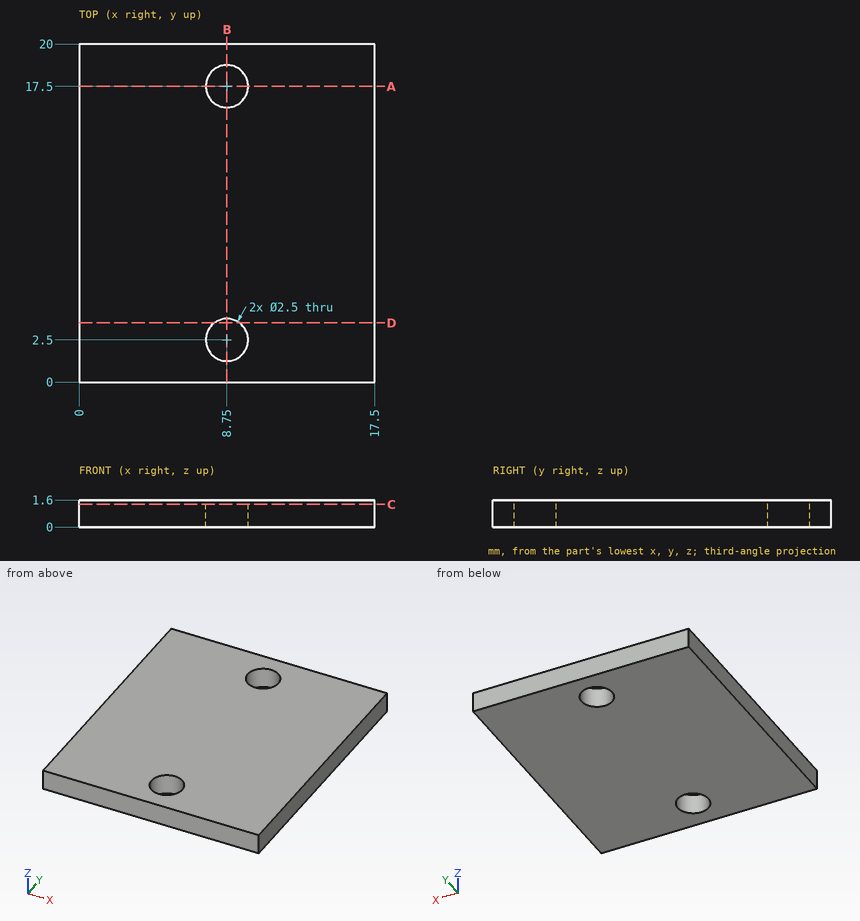
The drawing under review shows one solid part. Ordinate dimensions are in mm from its lowest x, y, z. Give positions to 0.01 mm unless a question says otherwise; leave off trailing zeros. Write each loop counter-clockwise with the first axis right and the second up, starting at its lowest first coordinate (ties: lowest second). Pieces come first, ordered by that corner, then holes.
1. Add section B-B, the plane x = 8.75. Write out the cut boundary in (y, z), plus the area to 3 significant figures.
2. Add section D-D, the plane y = 3.5. Write out the cut boundary in (x, z).
3. Wall thickness on L1, parallel to Y at x = 8.75, z = 0.75; L2, parallel to X at y = 17.5, z = 0.55; L3, parallel to Y at x = 8.25, z = 0.95: over which ranges is each line inside the solid? List them lowest first.
4. Add section C-C, the plane z = 1.35. Write out the cut boundary in (x, y).
5. Add section A-A, the plane y = 17.5. Write out the cut boundary in (x, z), plus the area to 3 significant figures.
Worked answers:
1. outline: (0, 0) - (1.25, 0) - (1.25, 1.6) - (0, 1.6) - close; (3.75, 0) - (16.25, 0) - (16.25, 1.6) - (3.75, 1.6) - close; (18.75, 0) - (20, 0) - (20, 1.6) - (18.75, 1.6) - close
1. area: 24.0 mm2
2. outline: (0, 0) - (8, 0) - (8, 1.6) - (0, 1.6) - close; (9.5, 0) - (17.5, 0) - (17.5, 1.6) - (9.5, 1.6) - close
3. L1: y = 0 to 1.25, 3.75 to 16.25, 18.75 to 20
3. L2: x = 0 to 7.5, 10 to 17.5
3. L3: y = 0 to 1.35, 3.65 to 16.35, 18.65 to 20
4. outline: (0, 0) - (17.5, 0) - (17.5, 20) - (0, 20) - close; hole circle Ø2.5 at (8.75, 2.5); hole circle Ø2.5 at (8.75, 17.5)
5. outline: (0, 0) - (7.5, 0) - (7.5, 1.6) - (0, 1.6) - close; (10, 0) - (17.5, 0) - (17.5, 1.6) - (10, 1.6) - close
5. area: 24.0 mm2
